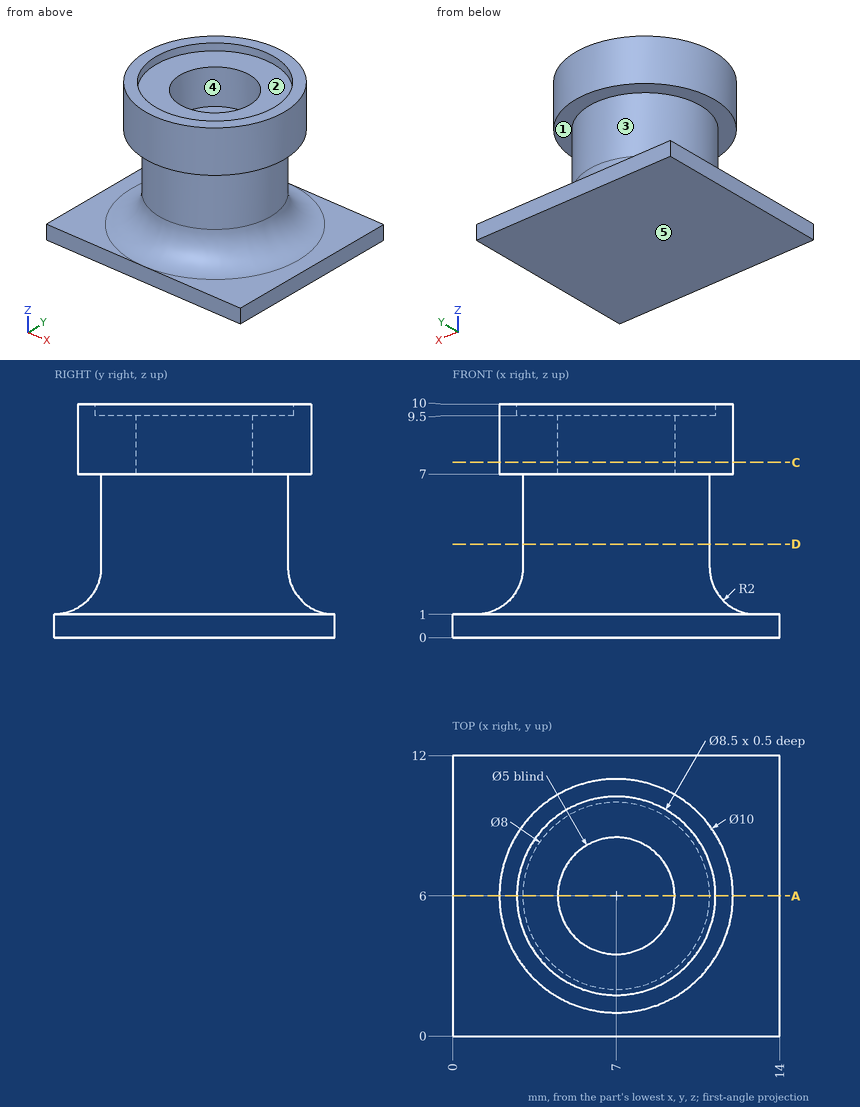
For this review, use the dimensioned drawing (mm, ordinates from the lowest corner) and the shaded views. A direction names the side the tool comes from. Coordinates: 2 decimals unless noted, no trailing zeros. Order: outer loops, then holes, each group sorted by start corner. A loop starts at its lowest first (then second) coordinate and runs counter-clockwise, first axis right, second up. Notation, with made-up numbers: (-9, -14) - (3, -14) arc R13 cw to (3, -8) - close; hole circle Ø8 at (3.5, 82). An arc over 180 degrees is marked (long way). Answer as a JSON object with one key per item and string values. Group by question number.
1. We need section A-A on y = 6. State the section outline as (x, z) points.
2. The part is to be moulded in two halves that separate along X. For the marked faces 1, 2 and 3, say which applies: pulls with the +X half, pulls with the -X half, needs draft (parallel to the pull), parting line crosses it, or undercut.
3. We need section D-D on z = 4. State the section outline as (x, y) points.
4. For the marked faces 4 and 5, list the 3-axis set-ups (+Z, -Z, +X, -X, +Y, -Y) from which the entire face can be reached by the end or side of a thin tool; tool diameter is ignored.
5. Clearance check with flat-ended pins moving along their axes: P1, Ø2.5, axis at x = 6, y = 7, coming from the +Z side; P2, Ø1.5, axis at y = 8, z = 2.5, coming from the -X side; P3, Ø1.5, axis at y = 8.5, z = 7.5, coming from the +X side. State where each tip first meets the part, or that it passes through.
6. We need section C-C on z = 7.5. State the section outline as (x, y) points.
7. For probe 1 along Y at (x, z) = (7, 9.75); probe 2 along Y at (x, z) = (7, 7.65); probe 3 along Z at (x, y) = (5.5, 3.75), list the stretches that pass through material, from the lowest coordinate up.
Final values:
{
 "1": {"outline": "(0, 0) - (14, 0) - (14, 1) - (13, 1) arc R2 cw to (11, 3) - (11, 7) - (12, 7) - (12, 10) - (11.25, 10) - (11.25, 9.5) - (9.5, 9.5) - (9.5, 7) - (4.5, 7) - (4.5, 9.5) - (2.75, 9.5) - (2.75, 10) - (2, 10) - (2, 7) - (3, 7) - (3, 3) arc R2 cw to (1, 1) - (0, 1) - close"},
 "2": {"face 1": "needs draft", "face 2": "undercut", "face 3": "parting line crosses it"},
 "3": {"outline": "circle Ø8 at (7, 6)"},
 "4": {"face 4": "+Z", "face 5": "-Z, +X, -X, +Y, -Y"},
 "5": {"P1": "z = 9.5", "P2": "x = 2.95", "P3": "x = 11.68"},
 "6": {"outline": "circle Ø10 at (7, 6); hole circle Ø5 at (7, 6)"},
 "7": {"probe 1": "1 to 1.75, 10.25 to 11", "probe 2": "1 to 3.5, 8.5 to 11", "probe 3": "0 to 9.5"}
}
